Verification items for the finished model (mm, model axes). A direction names the side the tool comes from. Round coordinates to 2 decimals unless told otherwise and drop trailing zeros. Write each loop counter-clockwise with the first axis right and the second up, starting at its lowest first coordinate (ties: lowest second). Pieces come first, ordered by that corner, then holes. Notation, with made-up numbers: M 59,-22.75 L 116,-22.75 A15 cw 116,-9.75 Z; hole C 77.5,42.25 d9. An arc over 180 degrees is marked long. Answer in a Markdown table with one row per item. Add a question column.
1. Material ranges on probe 1 along X at (y, z) = (-57, 49.5); probe 2 along Z at (x, y) = (-15.5, -65); probe 3 along Z at (x, y) = (-36, -12), recorded low to high.
2. Sectioned sample at C-C on y = -6. Record the cut outline in (x, z).
3. Draft check along Z on faces 1 (the cylindrical face through (-5.376, -56.8, 42.498)), 2 (the flat face through (-22, -25.4, 36)), 3 (the flat face through (-19, -46, 76.2)). Enter one of: pulls with the +Z half, pulls with the -Z half, needs draft (parallel to the pull), parting line crosses it, or undercut.
4. Sectioned sample at A-A on x = -29. Record the cut outline in (y, z), plus the area to 3 significant figures.
5. Sectioned sample at D-D on y = -30. Record the cut outline in (x, z), plus the area to 3 significant figures.
6. Sectioned sample at B-B on z = 63. Record the cut outline in (x, y).
7. Set-up check for faces 4 (the flat face through (-19, -76.2, 30)), 5 (the cylindrical face through (-29.065, -2.549, 57.417)): record each of +Z, -Z, +X, -X, +Y, -Y from which the full face is reachable in a straight line by a thin tool's end or side.
8. Go/stop test with flat-tipped pins: pin 1 Ø12 at (x, y) = (-21, -20.5) entering from +Z; pin 2 Ø3.5 at (x, z) = (-27, 36.5) entering from -Y. Record where each tip stops, or that it passes through.
```python
from build123d import *

# Parameters (mm, degrees)
F0_W     = 127
F0_H     = 76.2
F1_DEPTH = 76.2
F2_R     = 20.895154
F3_DEPTH = 38.1
F4_R     = 17.773402
F5_DEPTH = 50.8


with BuildPart() as f1:
    # F0 (on Front) → F1 (new body)
    with BuildSketch(Plane.XZ):
        with Locations((-18.322727, 38.1)):
            Rectangle(F0_W, F0_H)
    extrude(amount=F1_DEPTH)

    # F2 (on face) → F3 (cut)
    with BuildSketch(Plane.XY.offset(76.2)):
        with Locations((-26.344616, -23.265893)):
            Circle(F2_R)
    extrude(amount=-F3_DEPTH, mode=Mode.SUBTRACT)

    # F4 (on face) → F5 (cut)
    with BuildSketch(Plane.XZ.offset(76.2)):
        with Locations((-21.794144, 49.305573)):
            Circle(F4_R)
    extrude(amount=-F5_DEPTH, mode=Mode.SUBTRACT)


solid = f1.part
```
Geometry check:
| question | item | result |
|---|---|---|
| 1 | probe 1 | x = -81.82 to -39.57, -4.02 to 45.18 |
| 1 | probe 2 | z = 0 to 32.68, 65.93 to 76.2 |
| 1 | probe 3 | z = 0 to 38.1 |
| 2 | outline | M -81.82,0 L 45.18,0 L 45.18,76.2 L -14.58,76.2 L -14.58,38.1 L -38.11,38.1 L -38.11,76.2 L -81.82,76.2 Z |
| 3 | face 1 | undercut |
| 3 | face 2 | needs draft |
| 3 | face 3 | pulls with the +Z half |
| 4 | outline | M -76.2,0 L 0,0 L 0,76.2 L -2.54,76.2 L -2.54,38.1 L -25.4,38.1 L -25.4,33.06 L -76.2,33.06 Z; M -76.2,65.55 L -43.99,65.55 L -43.99,76.2 L -76.2,76.2 Z |
| 4 | area | 3,090 mm2 |
| 5 | outline | M -81.82,0 L 45.18,0 L 45.18,76.2 L -6.56,76.2 L -6.56,58.47 A17.77 cw -6.56,40.14 L -6.56,38.1 L -8,38.1 A17.77 cw -35.59,38.1 L -46.12,38.1 L -46.12,76.2 L -81.82,76.2 Z |
| 5 | area | 8,010 mm2 |
| 6 | outline | M -81.82,-76.2 L -33.12,-76.2 L -33.12,-43.03 A20.9 cw long -10.46,-36.85 L -10.46,-76.2 L 45.18,-76.2 L 45.18,0 L -81.82,0 Z |
| 7 | face 4 | +Z, -Z, +X, -X, -Y |
| 7 | face 5 | +Z |
| 8 | pin 1 | stops at z = 38.1 |
| 8 | pin 2 | stops at y = -25.4 |
